from build123d import *

# Parameters (mm, degrees)
SURFACE_EXTRUDE1_1_DEPTH = 600
THICKEN1_T1              = 2
SKETCH3_R                = 4
CUT_EXTRUDE1_DEPTH       = 2
SKETCH4_R                = 4
CUT_EXTRUDE2_DEPTH       = 2
LPATTERN1_COUNT          = 2
LPATTERN1_PITCH          = 560


with BuildPart() as body_1:
    # Surface-Extrude1: a surface, the sketch's curves swept straight by 600 mm
    with BuildLine(Plane(origin=(0, 0, 0), x_dir=(0, 0, -1), z_dir=(1, 0, 0)), mode=Mode.PRIVATE) as surface_extrude1_1_path:
        Line((0, 0), (-49.56534309, 49.56534309))
        ThreePointArc((-49.56534309, 49.56534309), (-53.830414293, 58.214051925), (-51.949122429, 67.671944808))
        Line((-51.949122429, 67.671944808), (264.050877571, 615))
        ThreePointArc((264.050877571, 615), (282.35214776, 633.301270189), (307.35214776, 640))
        Line((307.35214776, 640), (347.35214776, 640))
    surface_extrude1_1 = Shell.extrude(surface_extrude1_1_path.wire(), (1 * SURFACE_EXTRUDE1_1_DEPTH, 0 * SURFACE_EXTRUDE1_1_DEPTH, 0 * SURFACE_EXTRUDE1_1_DEPTH))
    add(Solid.thicken(surface_extrude1_1, THICKEN1_T1))

    # Sketch3 → Cut-Extrude1 (cut)
    with BuildSketch(Plane(origin=(0, -1.414213562, 1.414213562), x_dir=(1, 0, 0), z_dir=(0, -0.7071067811865517, 0.7071067811865434))):
        with Locations(Location((580, 33.095980422, 0), (0, 0, 270))):
            Circle(SKETCH3_R)
    cut_extrude1 = extrude(amount=-CUT_EXTRUDE1_DEPTH, mode=Mode.SUBTRACT)

    # Sketch4 → Cut-Extrude2 (cut)
    with BuildSketch(Plane(origin=(0, 642, 0), x_dir=(1, 0, 0), z_dir=(0, 1, 0))):
        with Locations(Location((580, 327.35214776, 0), (0, 0, 270))):
            Circle(SKETCH4_R)
    cut_extrude2 = extrude(amount=-CUT_EXTRUDE2_DEPTH, mode=Mode.SUBTRACT)

    # LPattern1: Cut-Extrude1, Cut-Extrude2 ×2
    with Locations(*[(-i * LPATTERN1_PITCH, 0, 0) for i in range(1, LPATTERN1_COUNT)]):
        add(cut_extrude1, mode=Mode.SUBTRACT)
        add(cut_extrude2, mode=Mode.SUBTRACT)


solid = body_1.part
Model file for the job. Use its own axes, mm. A direction names the side the tool comes from. Coordinates: 2 decimals unless noted, no trailing zeros. Order: outer loops, then holes, each group sorted by start corner. A loop starts at its lowest first (then second) coordinate and runs counter-clockwise, first axis right, second up. Notation, with made-up numbers: (57.25, 60) -> (91.25, 60) arc R22 cw to (91.25, 78) -> close; hole circle Ø6 at (-18, 37.5). An arc over 180 degrees is marked (long way). Return JSON: item names as keys, results as strings. Group by question number.
Item 1: Saw through at A-A on x = 182.5. Write the cut outline in (y, z).
Item 2: Wall check: line 1 along Y through (x, z) = (212.5, -313); line 2 along Z through (x, y) = (377.5, 485); line 3 along Y through (x, z) = (431, -109.5). Give the ranges that are in metal, low to high. Write a range as [from, to].
Item 3: Saw through at C-C on z = -251.5. Write the cut outline in (x, y), then the cut area to 3 significant figures.
Item 4: Tool access for faces 1 (the flat face through (296, 640, -327)), 2 (the flat face through (296, 642, -327)), 3 (the flat face through (295.8, 337.505, -103.839)): list every direction of +Z, -Z, +X, -X, +Y, -Y with a clear straight run to the whole face (end or side of a thin tool).
Item 5: Pull direction Y, two halves, no side cores. Call faces 4 (the flat face through (295.8, 23.02, 25.85)), 5 (the flat face through (296, 24, 24)), 6 (the cylindrical face through (295.8, 634.84, -281.02)): pulls with the +Y half, pulls with the -Y half, needs draft (parallel to the pull), parting line crosses it, or undercut.
Item 6: Flat gauge pins, fed straight in: P1, Ø5, axis at x = 314, y = 318.5, coming from the +Z side; P2, Ø2, axis at x = 359, z = -106, coming from the -Y side; P3, Ø6, axis at x = 357.5, y = 136, coming from the -Z side. Where does each tip first touch, or does it go through?
Item 7: Saw through at B-B on y = 506.5. Write the cut outline in (x, z), then the cut area to 3 significant figures.
Values found:
{
 "1": {"outline": "(-1.41, 1.41) -> (0, 0) -> (49.57, 49.57) arc R15 cw to (67.67, 51.95) -> (615, -264.05) arc R50 cw to (640, -307.35) -> (640, -347.35) -> (642, -347.35) -> (642, -307.35) arc R52 ccw to (616, -262.32) -> (68.67, 53.68) arc R17 ccw to (48.15, 50.98) -> close"},
 "2": {"line 1": "y = [640, 642]", "line 2": "z = [-189, -186.69]", "line 3": "y = [347.31, 351.31]"},
 "3": {"outline": "(0, 593.26) -> (600, 593.26) -> (600, 597.26) -> (0, 597.26) -> close", "area": "2,400 mm2"},
 "4": {"face 1": "-Z, +X, -X, -Y", "face 2": "+Z, -Z, +X, -X, +Y", "face 3": "-Z, +X, -X"},
 "5": {"face 4": "pulls with the -Y half", "face 5": "undercut", "face 6": "pulls with the +Y half"},
 "6": {"P1": "stops at z = -89.11", "P2": "stops at y = 339.52", "P3": "stops at z = 10.77"},
 "7": {"outline": "(0, -201.41) -> (600, -201.41) -> (600, -199.1) -> (0, -199.1) -> close", "area": "1,390 mm2"}
}
